Can you work these out from the model? Positions are in its coordinate system, mm. Face numbers are marked on the shaded views. Coordinates: 2 decimals unless noted, no trailing zeros. Order: outer loops, then holes, each group sorted by start corner. A loop starts at its lowest first (then second) coordinate and runs counter-clockwise, first axis right, second up. Notation, with made-up numbers: (35, 20) -> (90, 20) arc R27 cw to (90, 46) -> close; hole circle Ø10 at (32, -22). An arc over 180 degrees is marked (long way). Use a Markdown table: item, result. Add a question column.
1. Suppose I cut it at C-C, the plane x = -49. List the corners of the cut face in (y, z) for me.
2. Suppose I cut it at B-B, the plane y = 1.5. State how many separate pieces and enclosed holes the cut face has, then the cut area to 3 significant figures.
3. We'd pull the mould along X, two halves only. Please class the marked faces 1 and 2: pulls with the +X half, pulls with the -X half, needs draft (parallel to the pull), parting line crosses it, or undercut.
4. Suppose I cut it at A-A, the plane z = -16. List the corners of the cut face in (x, y) for me.
5. For pin 1 Ø4 at (x, z) = (-41.5, -31.5) entering from -Y; pin 2 Ø3.5 at (x, z) = (-246, -4) entering from +Y, each with a flat end and sliding along its axis, tell me the tip position at first contact or that it passes through.
6. If I drill on line 1 along X through (y, z) = (1.8, -29.9); line 2 along X through (y, z) = (1.8, -35.9); line 3 along X through (y, z) = (-1.85, -35.9), over which ranges is the centre line in solid material (lowest first)? Write a range as from..to.
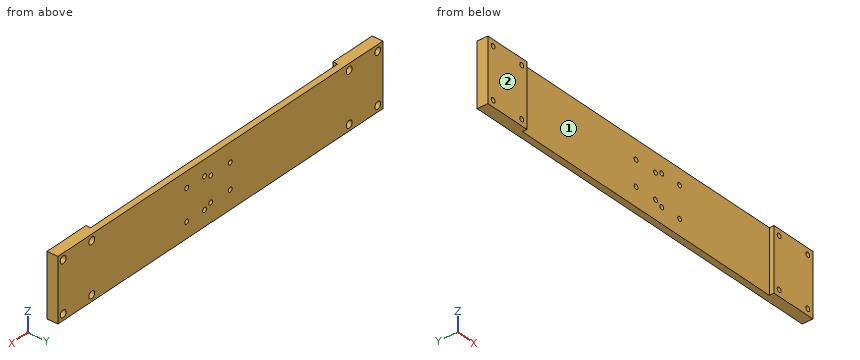
```python
from build123d import *
from build123d.topology import SkipClean

# Parameters (mm, degrees)
SKETCH_1_W          = 250
SKETCH_1_H          = 39.9
EXTRUDE_1_DEPTH     = 4
SKETCH_2_R          = 1.45
CUT_EXTRUDE_1_DEPTH = 12
SKETCH_3_R          = 1.45
CUT_EXTRUDE_2_DEPTH = 12
SKETCH_7_R          = 2.25
CUT_EXTRUDE_6_DEPTH = 20
SKETCH_8_W          = 30
SKETCH_8_H          = 39.9
SKETCH_8_R          = 2.25
EXTRUDE_2_DEPTH     = 1
SKETCH_9_W          = 30
SKETCH_9_H          = 39.9
EXTRUDE_3_DEPTH     = 2
SKETCH_10_R         = 1.5
CUT_EXTRUDE_7_DEPTH = 3


with BuildPart() as part:
    # Sketch 1 → Extrude 1 (new body)
    with BuildSketch(Plane(origin=(0, 0, 0), x_dir=(1, 0, 0), z_dir=(0, 1, 0))):
        with Locations((-125, 19.95)):
            Rectangle(SKETCH_1_W, SKETCH_1_H)
    extrude(amount=EXTRUDE_1_DEPTH)

    # Sketch 2 → Cut-Extrude 1 (cut)
    with BuildSketch(Plane(origin=(0, 4, 0), x_dir=(1, 0, 0), z_dir=(0, 1, 0))):
        with Locations(Location((-132.5, 27.95, 0), (0, 0, 270))):
            Circle(SKETCH_2_R)
        with Locations(Location((-117.5, 27.95, 0), (0, 0, 270))):
            Circle(SKETCH_2_R)
        with Locations(Location((-117.5, 11.95, 0), (0, 0, 270))):
            Circle(SKETCH_2_R)
        with Locations(Location((-132.5, 11.95, 0), (0, 0, 270))):
            Circle(SKETCH_2_R)
    extrude(amount=-CUT_EXTRUDE_1_DEPTH, mode=Mode.SUBTRACT)

    # Sketch 3 → Cut-Extrude 2 (cut)
    with BuildSketch(Plane(origin=(-275.091791604, 0, 148.847510468), x_dir=(-0.9999983055135633, 0, 0.0018409155336922224), z_dir=(0, -1, 0))):
        with Locations(Location((-162.633941367, 158.548383777, 0), (0, 0, 90.10547675))):
            Circle(SKETCH_3_R)
        with Locations(Location((-162.670575586, 178.448350057, 0), (0, 0, 90.10547675))):
            Circle(SKETCH_3_R)
        with Locations(Location((-176.383918068, 158.523071189, 0), (0, 0, 90.10547675))):
            Circle(SKETCH_3_R)
        with Locations(Location((-176.420552287, 178.423037468, 0), (0, 0, 90.10547675))):
            Circle(SKETCH_3_R)
    extrude(amount=-CUT_EXTRUDE_2_DEPTH, mode=Mode.SUBTRACT)

    # Sketch 7 → Cut-Extrude 6 (cut)
    with BuildSketch(Plane(origin=(0, 4, 0), x_dir=(1, 0, 0), z_dir=(0, 1, 0))):
        with Locations(Location((-246, 35.9, 0), (0, 0, 270))):
            Circle(SKETCH_7_R)
        with Locations(Location((-224, 35.9, 0), (0, 0, 270))):
            Circle(SKETCH_7_R)
        with Locations(Location((-224, 4, 0), (0, 0, 270))):
            Circle(SKETCH_7_R)
        with Locations(Location((-246, 4, 0), (0, 0, 270))):
            Circle(SKETCH_7_R)
        with Locations(Location((-4, 4, 0), (0, 0, 270))):
            Circle(SKETCH_7_R)
        with Locations(Location((-26, 4, 0), (0, 0, 270))):
            Circle(SKETCH_7_R)
        with Locations(Location((-26, 35.9, 0), (0, 0, 270))):
            Circle(SKETCH_7_R)
        with Locations(Location((-4, 35.9, 0), (0, 0, 270))):
            Circle(SKETCH_7_R)
    extrude(amount=-CUT_EXTRUDE_6_DEPTH, mode=Mode.SUBTRACT)

    # Sketch 8 → Extrude 2 (add)
    # profile 1 of 2: a face of its own
    with SkipClean():  # the faces are left unmerged after this step: merging them gives an invalid solid
        with BuildSketch(Plane.XZ):
            with Locations((-235, -19.95)):
                Rectangle(SKETCH_8_W, SKETCH_8_H)
            with Locations(Location((-224, -35.9, 0), (0, 0, 90))):
                Circle(SKETCH_8_R, mode=Mode.SUBTRACT)
            with Locations(Location((-246, -35.9, 0), (0, 0, 90))):
                Circle(SKETCH_8_R, mode=Mode.SUBTRACT)
            with Locations(Location((-224, -4, 0), (0, 0, 270))):
                Circle(SKETCH_8_R, mode=Mode.SUBTRACT)
            with Locations(Location((-246, -4, 0), (0, 0, 270))):
                Circle(SKETCH_8_R, mode=Mode.SUBTRACT)
        # profile 2 of 2: a face of its own
        with BuildSketch(Plane.XZ):
            with Locations((-15, -19.95)):
                Rectangle(SKETCH_8_W, SKETCH_8_H)
            with Locations(Location((-4, -35.9, 0), (0, 0, 270))):
                Circle(SKETCH_8_R, mode=Mode.SUBTRACT)
            with Locations(Location((-26, -35.9, 0), (0, 0, 270))):
                Circle(SKETCH_8_R, mode=Mode.SUBTRACT)
            with Locations(Location((-4, -4, 0), (0, 0, 90))):
                Circle(SKETCH_8_R, mode=Mode.SUBTRACT)
            with Locations(Location((-26, -4, 0), (0, 0, 90))):
                Circle(SKETCH_8_R, mode=Mode.SUBTRACT)
        extrude(amount=EXTRUDE_2_DEPTH)
    add(part.part.scale(1), mode=Mode.REPLACE)  # the faces are merged on a copy

    # Sketch 9 → Extrude 3 (add)
    with BuildSketch(Plane.XZ.offset(1)):
        with Locations((-15, -19.95)):
            Rectangle(SKETCH_9_W, SKETCH_9_H)
        with Locations((-235, -19.95)):
            Rectangle(SKETCH_9_W, SKETCH_9_H)
    extrude(amount=EXTRUDE_3_DEPTH)

    # Sketch 10 → Cut-Extrude 7 (cut)
    with BuildSketch(Plane(origin=(0, -1, 0), x_dir=(1, 0, 0), z_dir=(0, 1, 0))):
        with Locations(Location((-246, 35.9, 0), (0, 0, 270))):
            Circle(SKETCH_10_R)
        with Locations(Location((-246, 4, 0), (0, 0, 270))):
            Circle(SKETCH_10_R)
        with Locations(Location((-224, 35.9, 0), (0, 0, 270))):
            Circle(SKETCH_10_R)
        with Locations(Location((-224, 4, 0), (0, 0, 270))):
            Circle(SKETCH_10_R)
        with Locations(Location((-26, 35.9, 0), (0, 0, 270))):
            Circle(SKETCH_10_R)
        with Locations(Location((-26, 4, 0), (0, 0, 270))):
            Circle(SKETCH_10_R)
        with Locations(Location((-4, 35.9, 0), (0, 0, 270))):
            Circle(SKETCH_10_R)
        with Locations(Location((-4, 4, 0), (0, 0, 270))):
            Circle(SKETCH_10_R)
    extrude(amount=-CUT_EXTRUDE_7_DEPTH, mode=Mode.SUBTRACT)


solid = part.part
```
Worked out:
| question | item | result |
|---|---|---|
| 1 | outline | (0, -39.9) -> (4, -39.9) -> (4, 0) -> (0, 0) -> close |
| 2 | separate pieces | 1 |
| 2 | enclosed holes | 16 |
| 2 | area | 9,790 mm² |
| 3 | face 1 | undercut |
| 3 | face 2 | needs draft |
| 4 | outline | (-250, -3) -> (-220, -3) -> (-220, 0) -> (-30, 0) -> (-30, -3) -> (0, -3) -> (0, 4) -> (-250, 4) -> close |
| 5 | pin 1 | stops at y = 0 |
| 5 | pin 2 | stops at y = -1 |
| 6 | line 1 | x = -250..-114.2, -111.3..-100.45, -97.55..0 |
| 6 | line 2 | x = -250..-248.25, -243.75..-226.25, -221.75..-28.25, -23.75..-6.25, -1.75..0 |
| 6 | line 3 | x = -250..-247.5, -244.5..-225.5, -222.5..-220, -30..-27.5, -24.5..-5.5, -2.5..0 |
